Autodesk Fusion 360 part; units mm, degrees
sketch "Sketch1" plane through (0, 0, 0) normal (0, 0, 1) x (1, 0, 0)
  line L0 (-95, 25) -> (-38, 25)
  line L1 (-38, 25) -> (-38, 84.5)
  line L2 (-38, 84.5) -> (-95, 84.5)
  line L3 (-95, 84.5) -> (-95, 25)
  dimension "d1" = 57
  dimension "d2" = 59.5
extrude "Extrude1" add sketch "Sketch1" along normal blind 32
shell "Shell1" thickness 1 removed faces 1 at (-76, 64.6667, 32)
draft "Draft1" angle -18 neutral plane through (-38, 84.5, 0) pull (0, 1, 0) 1 faces at (-94.6667, 64.3333, 32)
sketch "Sketch4" plane through (0, 25, 0) normal (0, -1, 0) x (1, 0, 0)
  line L0 (-95, 0) -> (-38, 0)
  line L1 (-38, 0) -> (-38, 12.6673)
  line L2 (-38, 12.6673) -> (-95, 12.6673)
  line L3 (-95, 12.6673) -> (-95, 0)
  line L4 (-63.6, 12.35) -> (-69.4, 12.35)
  arc A0 (-69.4, 12.35) -> (-69.4, 5.65) centre (-69.4, 9) ccw
  line L5 (-69.4, 5.65) -> (-63.6, 5.65)
  arc A1 (-63.6, 5.65) -> (-63.6, 12.35) centre (-63.6, 9) ccw
  line L6 (-60.25, 9) -> (-72.75, 9) construction
  dimension "d15" = 12.5
  dimension "d16" = 6.7
extrude "Extrude4" cut sketch "Sketch4" against normal blind 1 contours L4 A0 L5 A1
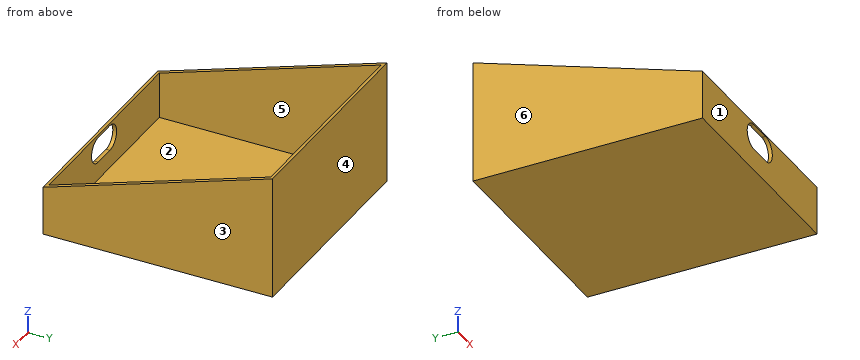
Input: part model. Units: mm. Frame: model coordinates. Face numbers are marked on the shaded views. A direction names the side the tool comes from. Give positions to 0.01 mm unless a question says otherwise; leave off trailing zeros. Order: outer loops, then holes, each group sorted by start corner. A loop starts at its lowest first (then second) coordinate and runs counter-clockwise, first axis right, second up. Notation, with made-up numbers: (32, -22.75) - (74, -22.75) arc R22 cw to (74, 2.25) - close; hole circle Ø8 at (21, 55.25). An arc over 180 degrees is marked (long way). Use a Markdown table: item, result.
(1) Access query for the marked faces 5 and 6. Directions: +Z, -Z, +X, -X, +Y, -Y. A direction counts if a zero-diameter tool reaches every point of the face in a straight line with its end or side. Return the directions, or none.
Computed values:
| item | result |
|---|---|
| face 5 | +Z |
| face 6 | +Z, -Z, -X, +Y, -Y |
(2) Section query D-D (y = 74). Output: boundary loops of the cut face in (x, z).
Computed values:
| item | result |
|---|---|
| outline | (-95, 0) - (-38, 0) - (-38, 28.59) - (-39, 28.59) - (-39, 1) - (-94, 1) - (-94, 28.59) - (-95, 28.59) - close |
(3) Section query A-A (x = -68). Output: boundary loops of the cut face in (y, z).
Computed values:
| item | result |
|---|---|
| outline | (25, 0) - (84.5, 0) - (84.5, 32) - (83.5, 31.68) - (83.5, 1) - (26, 1) - (26, 5.65) - (25, 5.65) - close; (25, 12.35) - (26, 12.35) - (26, 12.99) - (25, 12.67) - close |
(4) Section query C-C (x = -87.5). Output: boundary loops of the cut face in (y, z).
Computed values:
| item | result |
|---|---|
| outline | (25, 0) - (84.5, 0) - (84.5, 32) - (83.5, 31.68) - (83.5, 1) - (26, 1) - (26, 12.99) - (25, 12.67) - close |
(5) Section query B-B (z = 9). Output: boundary loops of the cut face in (x, y).
Computed values:
| item | result |
|---|---|
| outline | (-95, 25) - (-72.75, 25) - (-72.75, 26) - (-94, 26) - (-94, 83.5) - (-39, 83.5) - (-39, 26) - (-60.25, 26) - (-60.25, 25) - (-38, 25) - (-38, 84.5) - (-95, 84.5) - close |
(6) Line query: line 1 (X direction, y = 38, z = 5.5); line 2 (Y direction, x = -83, z = 2); line 3 (Z direction, x = -52.5, y = 66.5). Output: solid intervals per line, ascending. Write a range as from..to.
Computed values:
| item | result |
|---|---|
| line 1 | x = -95..-94, -39..-38 |
| line 2 | y = 25..26, 83.5..84.5 |
| line 3 | z = 0..1 |
(7) Pin query (flat end, axial travel): pin 1 (12 mm diameter, centred on x = -73, y = 45, fed in from -Z); pin 2 (12 mm diameter, centred on x = -45.5, y = 61.5, fed in from +Z); pin 3 (6 mm diameter, centred on x = -60, z = 26.5, fed in from -Y). Return the tip coordinate at first contact, or that it passes through.
Computed values:
| item | result |
|---|---|
| pin 1 | stops at z = 0 |
| pin 2 | stops at z = 1 |
| pin 3 | stops at y = 83.5 |
(8) Draft query along Y for the marked faces 1, 2, 3 and 4. Return one class per face: released by +Y, released by -Y, zero draft, split by the parting line, or undercut.
Computed values:
| item | result |
|---|---|
| face 1 | released by -Y |
| face 2 | undercut |
| face 3 | zero draft |
| face 4 | released by +Y |
